```python
from build123d import *

# Parameters (mm, degrees)
SKETCH_1_W          = 120
SKETCH_1_H          = 120
EXTRUDE_1_DEPTH     = 8
SKETCH_3_R          = 2.25
CUT_EXTRUDE_1_DEPTH = 8
SKETCH_4_R          = 4.4
CUT_EXTRUDE_2_DEPTH = 3
SKETCH_5_R          = 1.75
CUT_EXTRUDE_3_DEPTH = 8
SKETCH_6_R          = 2.9
CUT_EXTRUDE_4_DEPTH = 3
SKETCH_7_R          = 1.75
CUT_EXTRUDE_5_DEPTH = 8
SKETCH_8_R          = 2.9
CUT_EXTRUDE_6_DEPTH = 3
SKETCH_9_W          = 92
SKETCH_9_H          = 106
CUT_EXTRUDE_7_DEPTH = 4


with BuildPart() as part:
    # 草图1 → 凸台-拉伸1 (new body)
    with BuildSketch(Plane.XY):
        with Locations((4.838054616, 23.07265118)):
            Rectangle(SKETCH_1_W, SKETCH_1_H)
    extrude(amount=EXTRUDE_1_DEPTH)

    # 草图3 → 切除-拉伸1 (cut)
    with BuildSketch(Plane.XY.offset(8)):
        with Locations((4.838054616, 77.454324244)):
            Circle(SKETCH_3_R)
    extrude(amount=-CUT_EXTRUDE_1_DEPTH, mode=Mode.SUBTRACT)

    # 草图4 → 切除-拉伸2 (cut)
    with BuildSketch(Plane.XY.offset(8)):
        with Locations((4.838054616, 77.454324244)):
            Circle(SKETCH_4_R)
    extrude(amount=-CUT_EXTRUDE_2_DEPTH, mode=Mode.SUBTRACT)

    # 草图5 → 切除-拉伸3 (cut)
    with BuildSketch(Plane.XY.offset(8)):
        with Locations((57.34, 31.45)):
            Circle(SKETCH_5_R)
    extrude(amount=-CUT_EXTRUDE_3_DEPTH, mode=Mode.SUBTRACT)

    # 草图6 → 切除-拉伸4 (cut)
    with BuildSketch(Plane.XY.offset(8)):
        with Locations((57.34, 31.45)):
            Circle(SKETCH_6_R)
    extrude(amount=-CUT_EXTRUDE_4_DEPTH, mode=Mode.SUBTRACT)

    # 草图7 → 切除-拉伸5 (cut)
    with BuildSketch(Plane.XY.offset(8)):
        with Locations((-47.66, 31.45)):
            Circle(SKETCH_7_R)
    extrude(amount=-CUT_EXTRUDE_5_DEPTH, mode=Mode.SUBTRACT)

    # 草图8 → 切除-拉伸6 (cut)
    with BuildSketch(Plane.XY.offset(8)):
        with Locations((-47.66, 31.45)):
            Circle(SKETCH_8_R)
    extrude(amount=-CUT_EXTRUDE_6_DEPTH, mode=Mode.SUBTRACT)

    # 草图9 → 切除-拉伸7 (cut)
    with BuildSketch(Plane.XY.offset(8)):
        with Locations((6.215593236, 17.526521265)):
            Rectangle(SKETCH_9_W, SKETCH_9_H)
    extrude(amount=-CUT_EXTRUDE_7_DEPTH, mode=Mode.SUBTRACT)


solid = part.part
```
Geometry: final body of the model. Coordinates: model frame, mm. A direction names the side the tool comes from. Round coordinates to 2 decimals unless told otherwise and drop trailing zeros. Loops run counter-clockwise (first coordinate to the right, second up) from the corner with the lowest first, then second, coordinate; pieces in that order, holes last.
Item 1: Section B-B, the plane y = 20.5. Output: boundary loops of the cut face in (x, z), plus the area to 3 significant figures.
Checked values:
outline: (-55.16, 0) - (64.84, 0) - (64.84, 8) - (52.22, 8) - (52.22, 4) - (-39.78, 4) - (-39.78, 8) - (-55.16, 8) - close
area: 592 mm2
Item 2: Reachability of faces 4 (the flat face through (0, 72, 8)), 5 (the flat face through (52.216, 17, 6)) from +Z, -Z, +X, -X, +Y, -Y: full face, straight path, thin tool, end or side. Return the list, or none.
Checked values:
face 4: +Z, +X, -X, +Y, -Y
face 5: +Z
Item 3: Mould query, pull axis Y, two halves, no side actions, for faces 1 (the flat face through (-46, 30, 5)), 2 (the flat face through (-55.162, 22, 4)), 3 (the flat face through (4, -36.927, 4)). Classes: released by +Y, released by -Y, zero draft, split by the parting line, or undercut.
Checked values:
face 1: undercut
face 2: zero draft
face 3: released by -Y
Item 4: Section A-A, the plane x = 57.34. Output: boundary loops of the cut face in (y, z), plus the area to 3 significant figures.
Checked values:
outline: (-36.93, 0) - (29.7, 0) - (29.7, 5) - (28.55, 5) - (28.55, 8) - (-36.93, 8) - close; (33.2, 0) - (83.07, 0) - (83.07, 8) - (34.35, 8) - (34.35, 5) - (33.2, 5) - close
area: 925 mm2
Item 5: Line query: L1, parallel to Y at x = -12, z = 5.5; L2, parallel to X at y = 43.5, z = 5; L3, parallel to Y at x = -47.66, z = 1.8. Output: solid intervals per line, ascending.
Checked values:
L1: y = -36.93 to -35.47, 70.53 to 83.07
L2: x = -55.16 to -39.78, 52.22 to 64.84
L3: y = -36.93 to 29.7, 33.2 to 83.07
Item 6: Contact query for flat-ended pins moving along their axis: P1, Ø3, axis at x = -48, y = 30.5, coming from the +Z side; P2, Ø2, axis at x = 57.34, y = 31.45, coming from the -Z side (1 decimal); P3, Ø6, axis at x = 44.5, y = 26.5, coming from the +Z side; P4, Ø9.5, axis at x = 3, y = 76.5, coming from the +Z side. Output: stop coordinate, or through.
Checked values:
P1: stops at z = 5
P2: passes through
P3: stops at z = 4
P4: stops at z = 8
Item 7: Section C-C, the plane x = 12.5. Output: boundary loops of the cut face in (y, z), plus the area to 3 significant figures.
Checked values:
outline: (-36.93, 0) - (83.07, 0) - (83.07, 8) - (70.53, 8) - (70.53, 4) - (-35.47, 4) - (-35.47, 8) - (-36.93, 8) - close
area: 536 mm2
